Autodesk Inventor part; units mm, degrees
ref_plane "YZ Plane" through (0, 0, 0) normal (1, 0, 0) x (0, 1, 0)
ref_plane "XZ Plane" through (0, 0, 0) normal (0, 1, 0) x (-1, 0, 0)
ref_plane "XY Plane" through (0, 0, 0) normal (0, 0, 1) x (1, 0, 0)
sketch "Sketch1" plane through (0, 0, 0) normal (0, 1, 0) x (-1, 0, 0)
  line L0 (-10.0497, 12.7691) -> (-22.4997, 12.7691)
  line L1 (-22.4997, 12.7691) -> (-22.4997, -25.2309)
  line L2 (-22.4997, -25.2309) -> (-10.0497, -25.2309)
  line L3 (-10.0497, -25.2309) -> (-10.0497, 12.7691)
  dimension "d0" = 12.45
  dimension "d1" = 38
extrude "Extrusion1" add sketch "Sketch1" along normal blind 46.3
sketch "Sketch2" plane through (0, 46.3, 0) normal (0, 1, 0) x (1, 0, 0)
  line L0 (13.1497, -12.7691) -> (13.1497, 21.7309)
  line L1 (13.1497, 21.7309) -> (22.4997, 21.7309)
  line L2 (22.4997, 21.7309) -> (22.4997, 25.2309)
  line L3 (22.4997, 25.2309) -> (10.0497, 25.2309)
  line L4 (10.0497, 25.2309) -> (10.0497, -12.7691)
  line L5 (10.0497, 25.2309) -> (10.0497, -12.7691)
  line L6 (10.0497, -12.7691) -> (13.1497, -12.7691)
  line L7 (13.1497, 21.7309) -> (22.4997, 21.7309)
  point P0 (0, 0)
  point P1 (22.4997, -12.7691)
  point P2 (17.8247, -12.7691)
  point P3 (17.8247, 21.7309)
extrude "Extrusion2" cut sketch "Sketch2" against normal blind 2
sketch "Sketch3" plane through (0, 44.3, 0) normal (0, 1, 0) x (1, 0, 0)
  line L0 (22.4997, -12.7691) -> (22.4997, 25.2309)
  line L1 (13.1497, 21.7309) -> (13.1497, -12.7691)
  line L2 (22.4997, 21.7309) -> (13.1497, 21.7309)
  line L3 (13.1497, 21.7309) -> (13.1497, 25.2309)
  line L4 (22.4997, 25.2309) -> (10.0497, 25.2309)
  line L5 (22.4997, 25.2309) -> (22.4997, 21.7309)
  point P0 (0, 0)
extrude "Extrusion3" cut sketch "Sketch3" against normal blind 44.8625
sketch "Sketch5" plane through (0, 0, 0) normal (0, -1, 0) x (1, 0, 0)
  line L0 (10.0497, -25.2309) -> (10.0497, 12.7691)
  line L1 (13.1497, -25.2309) -> (10.0497, -25.2309)
  line L2 (10.0497, -25.2309) -> (13.1497, -25.2309)
  line L3 (13.1497, -21.7309) -> (13.1497, 12.7691)
  line L4 (13.1497, -25.2309) -> (13.1497, 12.7691)
  line L5 (13.1497, 12.7691) -> (10.0497, 12.7691)
  line L6 (10.0497, 12.7691) -> (10.0497, -25.2309)
  point P0 (0, 0)
extrude "Extrusion4" cut sketch "Sketch5" against normal blind 2
properties part number "MiniBB_SD_PD"
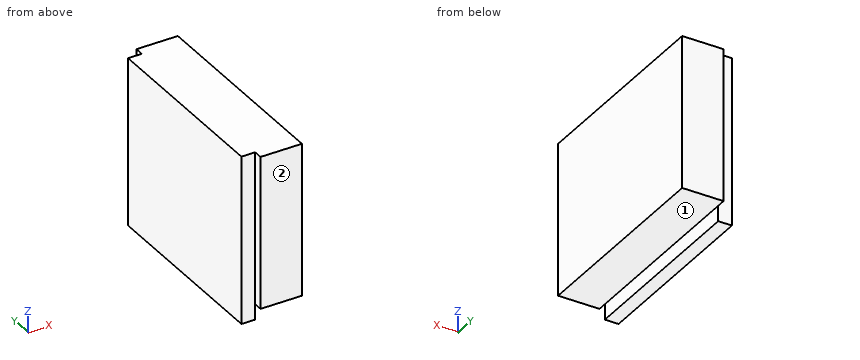
Verification items for the finished model (mm, model axes). Face numbers are marked on the shaded views. A direction names the side the tool comes from. Coordinates: 2 decimals unless noted, no trailing zeros. Write each loop counter-clockwise with the first axis right and the second up, starting at its lowest first coordinate (ties: lowest second). Pieces come first, ordered by that corner, then holes. Notation, with made-up numbers: M -30,66.25 L -17,66.25 A34 cw -17,101.25 Z; hole C -19,47.25 d5. An arc over 180 degrees is marked long. One line per question, with ' | ' between items.
1) Sectioned sample at C-C on x = 14.25. Record the cut outline in (y, z).
Solutions:
outline: M 0,-21.73 L 46.3,-21.73 L 46.3,12.77 L 0,12.77 Z
2) Sectioned sample at A-A on y = 43. Record the cut outline in (x, z), then the cut area to 3 significant figures.
Solutions:
outline: M 10.05,-25.23 L 13.15,-25.23 L 13.15,-21.73 L 22.5,-21.73 L 22.5,12.77 L 10.05,12.77 Z | area: 440 mm^2
3) Sectioned sample at D-D on z = -23. Record the cut outline in (x, y), then the cut area to 3 significant figures.
Solutions:
outline: M 10.05,2 L 13.15,2 L 13.15,44.3 L 10.05,44.3 Z | area: 131 mm^2
4) Material ranges on L1, parallel to Z at x = 18, y = 44.5; L2, parallel to Y at x = 10.5, z = -11.5; L3, parallel to X at y = 44.5, z = 7.5, recorded low to high.
Solutions:
L1: -21.73 to 12.77 | L2: 2 to 44.3 | L3: 13.15 to 22.5
5) Depth check by flat-ended pin: pin 1 Ø3 at (y, z) = (13, -24) entering from +X; pin 2 Ø1.6 at (y, z) = (1.5, -4.5) entering from -X; pin 3 Ø3.5 at (x, z) = (11, -4.5) entering from -Y; pin 4 Ø1.6 at (y, z) = (45.5, -7) entering from -X. Enter the tip coordinate at first touch or a pass-through.
Solutions:
pin 1: x = 13.15 | pin 2: x = 10.05 | pin 3: y = 2 | pin 4: x = 13.15
6) Sectioned sample at B-B on z = -13. Record the cut outline in (x, y), then the cut area to 3 significant figures.
Solutions:
outline: M 10.05,2 L 13.15,2 L 13.15,0 L 22.5,0 L 22.5,46.3 L 13.15,46.3 L 13.15,44.3 L 10.05,44.3 Z | area: 564 mm^2
7) Access from +Z, -Z, +X, -X, +Y, -Y to the whole of each face (thin tool, end or side, straight path). Record for the marked faces 1 and 2.
Solutions:
face 1: -Z, +X, +Y, -Y | face 2: +Z, -Z, +X, -X, -Y
